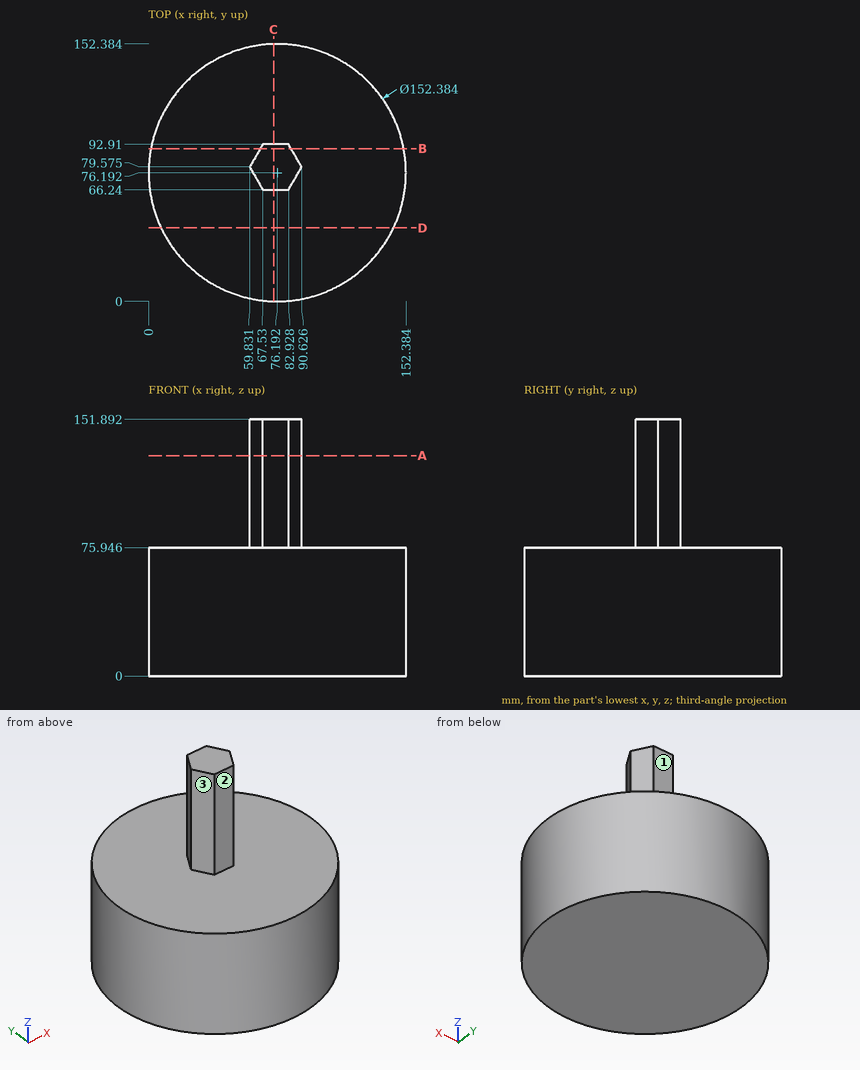
Job drawing, mm, ordinate dimensions from the low corner. One solid piece. A direction names the side the tool comes from. Round coordinates to 2 decimals unless told otherwise and drop trailing zeros. Write each loop counter-clockwise with the first axis right and the second up, starting at its lowest first coordinate (ties: lowest second). Pieces come first, ordered by that corner, then holes.
1) Band-saw the part on B-B, the plane y = 90.5. List the corners of the cut face in (x, z) (1 decimal).
2) Band-saw the part on D-D, the plane y = 43.5. List the corners of the cut face in (x, z), and give its area (3 significant figures).
3) Band-saw the part on A-A, the plane z = 130.5. List the corners of the cut face in (x, y) (1 decimal), and give its area (3 significant figures).
4) Drill centre lines: probe 1 along Z at (x, y) = (37, 140.5); probe 2 along X at (y, z) = (74.5, 28.5) (1 decimal); probe 3 along X at (y, z) = (120, 23) (1 decimal). Where is each one in solid material? Low to high.
5) Band-saw the part on C-C, the plane x = 74. List the corners of the cut face in (y, z), and give its area (3 significant figures).
6) 3-axis set-ups, long thin cutter, end or side, ignore diameter. For the marked faces 1, 2 and 3: which of +Z, -Z, +X, -X, +Y, -Y reach the whole face in a straight line?
7) Pin check, flat tips, straight feed: pin 1 (12 mm diameter, centred on y = 25, z = 22, fed in from +X) (1 decimal); pin 2 (8 mm diameter, centred on x = 85, z = 35.5, fed in from -Y); pin 3 (10 mm diameter, centred on x = 135.5, z = 34.5, fed in from -Y). Stop position of each tip, or through.
Ans:
1. outline: (1.4, 0) - (151, 0) - (151, 75.9) - (84.3, 75.9) - (84.3, 151.9) - (66.1, 151.9) - (66.1, 75.9) - (1.4, 75.9) - close
2. outline: (7.37, 0) - (145.01, 0) - (145.01, 75.95) - (7.37, 75.95) - close
2. area: 10,500 mm2
3. outline: (59.8, 79.6) - (67.5, 66.2) - (82.9, 66.2) - (90.6, 79.6) - (82.9, 92.9) - (67.5, 92.9) - close
3. area: 616 mm2
4. probe 1: z = 0 to 75.95
4. probe 2: x = 0 to 152.4
4. probe 3: x = 13.9 to 138.5
5. outline: (0.03, 0) - (152.35, 0) - (152.35, 75.95) - (92.91, 75.95) - (92.91, 151.89) - (66.24, 151.89) - (66.24, 75.95) - (0.03, 75.95) - close
5. area: 13,600 mm2
6. face 1: +Z, +X, -X, +Y
6. face 2: +Z, +X, -X, -Y
6. face 3: +Z, -X, -Y
7. pin 1: stops at x = 137.5
7. pin 2: stops at y = 0.15
7. pin 3: stops at y = 22.75
